from build123d import *

# Parameters (mm, degrees)
SKETCH1_W               = 45
SKETCH1_H               = 20
BOSS_EXTRUDE1_DEPTH     = 1.5
SKETCH2_W               = 15
SKETCH2_H               = 3
BOSS_EXTRUDE2_DEPTH     = 1.5
CUT_EXTRUDE1_DEPTH      = 27.02883017
CUT_EXTRUDE1_DEPTH_BACK = 27.02883017


with BuildPart() as part:
    # Sketch1 → Boss-Extrude1 (new, symmetric)
    with BuildSketch(Plane(origin=(0, 0, 0), x_dir=(1, 0, 0), z_dir=(0, 1, 0))):
        Rectangle(SKETCH1_W, SKETCH1_H)
    extrude(amount=BOSS_EXTRUDE1_DEPTH, both=True)

    # Sketch2 → Boss-Extrude2 (add, symmetric)
    with BuildSketch(Plane(origin=(0, 0, 0), x_dir=(1, 0, 0), z_dir=(0, 1, 0))):
        with Locations((0, -11.5)):
            Rectangle(SKETCH2_W, SKETCH2_H)
        with Locations((0, 11.5)):
            Rectangle(SKETCH2_W, SKETCH2_H)
    extrude(amount=BOSS_EXTRUDE2_DEPTH, both=True)

    # Sketch3 → Cut-Extrude1 (cut, two sides: drawn at the far end of the back side and taken through both)
    with BuildSketch(Plane(origin=(0, 0, 0), x_dir=(1, 0, 0), z_dir=(0, 1, 0)).offset(-CUT_EXTRUDE1_DEPTH_BACK)):
        with BuildLine():
            Line((-1.5, -13), (1.5, -13))
            Line((1.5, -13), (1.5, -9))
            Line((1.5, -9), (2.85, -9))
            Line((2.85, -9), (2.85, -6.73))
            Line((2.85, -6.73), (1.5, -6.73))
            Line((1.5, -6.73), (1.5, -2))
            ThreePointArc((1.5, -2), (1.207106781, -1.292893219), (0.5, -1))
            Line((0.5, -1), (-0.5, -1))
            ThreePointArc((-0.5, -1), (-1.207106781, -1.292893219), (-1.5, -2))
            Line((-1.5, -2), (-1.5, -6.73))
            Line((-1.5, -6.73), (-2.85, -6.73))
            Line((-2.85, -6.73), (-2.85, -9))
            Line((-2.85, -9), (-1.5, -9))
            Line((-1.5, -9), (-1.5, -13))
        make_face()
    extrude(amount=CUT_EXTRUDE1_DEPTH + CUT_EXTRUDE1_DEPTH_BACK, mode=Mode.SUBTRACT)


solid = part.part
Read the model definition and answer for the solid it produces. Units are mm, in the model's axes. A direction names the side the tool comes from. Coordinates: 2 decimals unless noted, no trailing zeros. Loops run counter-clockwise (first coordinate to the right, second up) from the corner with the lowest first, then second, coordinate; pieces in that order, holes last.
Q1. The mould has two halves that part along X. Classify faces 1 (the face through (2.85, 0, 8)), 2 (the face through (15, 0, -10)), 3 (the face through (22.5, 0, 0)), 4 (the face through (-2, 0, 9)): +X half, -X half, draft (parallel to the pull), parting line (faces both ways), or undercut.
Q2. Each of these flat-tipped pins is pushed along its axis until it touches: pin 1 Ø0.9 at (x, y) = (13.5, 0) entering from -Z; pin 2 Ø1.5 at (y, z) = (-0.5, -11) entering from +X. Where does it stop, or does it pass through?
Q3. The part is cut by section C-C on y = -0.45. Write down the section's boundary in (x, z), and give its area (3 significant figures).
Q4. The part is cut by section B-B on x = 2. Write down the section's boundary in (y, z).
Q5. The part is cut by section A-A on z = 11.5. Write down the section's boundary in (x, y), and give its area (3 significant figures).
Q6. The part is cut by section D-D on x = 10. Write down the section's boundary in (y, z).
Q7. Which of the six approach directions +Z, -Z, +X, -X, +Y, -Y give full straight-line access (tool end or side, diameter ignored) to faces 5 (the face through (7.5, 0, 12)), 6 (the face through (2, 0, 9)), 7 (the face through (-1.5, 0, 11))?
Q8. Consider probe 1 along X at (y, z) = (-0.6, 4.5); probe 2 along X at (y, z) = (0.75, 10.5); probe 3 along Z at (x, y) = (-2, 0.7). Determine where each line is inside the solid, lowest interval first.
Results below:
1. face 1: undercut
1. face 2: draft
1. face 3: +X half
1. face 4: undercut
2. pin 1: stops at z = -10
2. pin 2: stops at x = 7.5
3. outline: (-22.5, -10) - (-7.5, -10) - (-7.5, -13) - (7.5, -13) - (7.5, -10) - (22.5, -10) - (22.5, 10) - (7.5, 10) - (7.5, 13) - (1.5, 13) - (1.5, 9) - (2.85, 9) - (2.85, 6.73) - (1.5, 6.73) - (1.5, 2) arc R1 cw to (0.5, 1) - (-0.5, 1) arc R1 cw to (-1.5, 2) - (-1.5, 6.73) - (-2.85, 6.73) - (-2.85, 9) - (-1.5, 9) - (-1.5, 13) - (-7.5, 13) - (-7.5, 10) - (-22.5, 10) - close
3. area: 948 mm2
4. outline: (-1.5, -13) - (1.5, -13) - (1.5, 6.73) - (-1.5, 6.73) - close; (-1.5, 9) - (1.5, 9) - (1.5, 13) - (-1.5, 13) - close
5. outline: (-7.5, -1.5) - (-1.5, -1.5) - (-1.5, 1.5) - (-7.5, 1.5) - close; (1.5, -1.5) - (7.5, -1.5) - (7.5, 1.5) - (1.5, 1.5) - close
5. area: 36.0 mm2
6. outline: (-1.5, -10) - (1.5, -10) - (1.5, 10) - (-1.5, 10) - close
7. face 5: +Z, +X, +Y, -Y
7. face 6: +Y, -Y
7. face 7: +Z, +Y, -Y
8. probe 1: x = -22.5 to -1.5, 1.5 to 22.5
8. probe 2: x = -7.5 to -1.5, 1.5 to 7.5
8. probe 3: z = -13 to 6.73, 9 to 13
